Could you check a few things on this model? Use its own coordinates, in mm. A direction names the side the tool comes from. Give positions to 0.01 mm unless a question says otherwise; leave off trailing zeros. Order: outer loops, then holes, each group sorted by start corner. A loop starts at its lowest first (then second) coordinate and runs counter-clockwise, first axis right, second up.
(1) Will these pins go through, and if not, where does the flat tip stop? pin 1 (10 mm diameter, centred on x = -18, y = -38, fed in from +Z); pin 2 (2 mm diameter, centred on x = 14.5, z = 20.5, fed in from +Y); pin 3 (12 mm diameter, centred on x = 15, y = 17, fed in from -Z).
(2) On a 3-axis mill with a long thin cutter (end or side, diameter ignored), from which of +Z, -Z, +X, -X, +Y, -Y can I reach the whole of each face in a straight line? I mean faces 5 (the flat face through (40.926, -13, 13)), 6 (the flat face through (-40.074, -13, 22)), 7 (the flat face through (-38, -1.008, 17)), 8 (the flat face through (18.926, 27, 14)), 9 (the flat face through (2, -12, 27)). Say none if no direction works.
(3) If I drill on probe 1 along X at (y, z) = (-23, 36.5); probe 2 along X at (y, z) = (-33, 14.5); probe 3 along Y at (x, z) = (0, 32), over which ranges is the centre line in solid material (lowest first)?
(4) If we mould it in two halves opening along Y, with no side actions, what happens to faces 1 (the flat face through (16.926, 27, 14)), 2 (the cylindrical face through (45.02, 28.14, 22.82)), 3 (the flat face through (-9, 23.992, 13)), 4 (the flat face through (2, -51.008, 36))? For each: released by +Y, released by -Y, zero draft, split by the parting line, or undercut.
(5) Imagine slicing it at A-A, the plane x = -2. Write out the boundary of the cut face in (y, z), then the cut area to 3 significant figures.
(6) Imagine slicing it at C-C, the plane y = -26. Write out the boundary of the cut face in (x, z).
(7) Imagine slicing it at B-B, the plane y = 13. Write out the boundary of the cut face in (x, z), then the cut area to 3 significant figures.
(8) Imagine slicing it at D-D, the plane x = -15. Write out the boundary of the cut face in (y, z), then the cut area to 3 significant figures.
from build123d import *

# Parameters (mm, degrees)
ESQUISSE1_W             = 86
ESQUISSE1_H             = 83
BOSS_EXTRU_1_DEPTH      = 45
ESQUISSE2_W             = 82
ESQUISSE2_H             = 79
ENL_V_MAT_EXTRU_1_DEPTH = 3
ESQUISSE3_W             = 76
ESQUISSE3_H             = 73
ENL_V_MAT_EXTRU_2_DEPTH = 20
ESQUISSE5_W             = 80
ESQUISSE5_H             = 77
ENL_V_MAT_EXTRU_3_DEPTH = 18
ESQUISSE7_W             = 20
ESQUISSE7_H             = 16
ENL_V_MAT_EXTRU_4_DEPTH = 18
ESQUISSE8_W             = 20
ESQUISSE8_H             = 16
ENL_V_MAT_EXTRU_5_DEPTH = 18
ESQUISSE10_W            = 10
ESQUISSE10_H            = 25
ENL_V_MAT_EXTRU_6_DEPTH = 18
ESQUISSE12_R            = 0.5
ENL_V_MAT_EXTRU_9_DEPTH = 18
CONG_2_R                = 3


with BuildPart() as part:
    # Esquisse1 → Boss.-Extru.1 (new body)
    with BuildSketch(Plane.XY):
        with Locations((2.925773196, -12.508247423)):
            Rectangle(ESQUISSE1_W, ESQUISSE1_H)
    extrude(amount=BOSS_EXTRU_1_DEPTH)

    # Esquisse2 → Enlèv. mat.-Extru.1 (cut)
    with BuildSketch(Plane(origin=(0, 0, 0), x_dir=(-1, 0, 0), z_dir=(0, 0, -1))):
        with Locations((-2.925773196, -12.508247423)):
            Rectangle(ESQUISSE2_W, ESQUISSE2_H)
    extrude(amount=-ENL_V_MAT_EXTRU_1_DEPTH, mode=Mode.SUBTRACT)

    # Esquisse3 → Enlèv. mat.-Extru.2 (cut)
    with BuildSketch(Plane(origin=(0, 0, 3), x_dir=(-1, 0, 0), z_dir=(0, 0, -1))):
        with Locations((-2.925773196, -12.508247423)):
            Rectangle(ESQUISSE3_W, ESQUISSE3_H)
    extrude(amount=-ENL_V_MAT_EXTRU_2_DEPTH, mode=Mode.SUBTRACT)

    # Esquisse5 → Enlèv. mat.-Extru.3 (cut)
    with BuildSketch(Plane.XY.offset(45)):
        with Locations((2.925773196, -12.508247423)):
            Rectangle(ESQUISSE5_W, ESQUISSE5_H)
    extrude(amount=-ENL_V_MAT_EXTRU_3_DEPTH, mode=Mode.SUBTRACT)

    # Esquisse7 → Enlèv. mat.-Extru.4 (cut)
    with BuildSketch(Plane(origin=(0, 28.991752577, 0), x_dir=(1, 0, 0), z_dir=(0, 1, 0))):
        with Locations((28.925773196, -14)):
            Rectangle(ESQUISSE7_W, ESQUISSE7_H)
    extrude(amount=-ENL_V_MAT_EXTRU_4_DEPTH, mode=Mode.SUBTRACT)

    # Esquisse8 → Enlèv. mat.-Extru.5 (cut)
    with BuildSketch(Plane(origin=(0, 28.991752577, 0), x_dir=(1, 0, 0), z_dir=(0, 1, 0))):
        with Locations((6.925773196, -14)):
            Rectangle(ESQUISSE8_W, ESQUISSE8_H)
    extrude(amount=-ENL_V_MAT_EXTRU_5_DEPTH, mode=Mode.SUBTRACT)

    # Esquisse10 → Enlèv. mat.-Extru.6 (cut)
    with BuildSketch(Plane.ZY.offset(40.074226804)):
        with Locations((17, 11.491752577)):
            Rectangle(ESQUISSE10_W, ESQUISSE10_H)
    extrude(amount=-ENL_V_MAT_EXTRU_6_DEPTH, mode=Mode.SUBTRACT)

    # Esquisse12 → Enlèv. mat.-Extru.9 (cut)
    with BuildSketch(Plane.ZY.offset(40.074226804)):
        with Locations((29, 3.991752577)):
            Circle(ESQUISSE12_R)
    extrude(amount=-ENL_V_MAT_EXTRU_9_DEPTH, mode=Mode.SUBTRACT)

    # Congé2
    cong_2_edges = [part.edges().sort_by_distance(p)[0] for p in [
        (-40.074226804, 28.991752577, 22.5),
        (45.925773196, 28.991752577, 22.5),
        (45.925773196, -54.008247423, 22.5),
        (-40.074226804, -54.008247423, 22.5),
    ]]
    fillet(cong_2_edges, radius=CONG_2_R)


solid = part.part
Answer block:
1. pin 1: stops at z = 27
1. pin 2: stops at y = -49.01
1. pin 3: stops at z = 23
2. face 5: -Z
2. face 6: +Z, -Z, -X, +Y, -Y
2. face 7: -X
2. face 8: +Y
2. face 9: +Z
3. probe 1: x = -40.07 to -37.07, 42.93 to 45.93
3. probe 2: x = -40.07 to -35.07, 40.93 to 45.93
3. probe 3: y = -54.01 to -51.01, 25.99 to 28.99
4. face 1: zero draft
4. face 2: released by +Y
4. face 3: undercut
4. face 4: undercut
5. outline: (-54.01, 0) - (-52.01, 0) - (-52.01, 3) - (-49.01, 3) - (-49.01, 23) - (23.99, 23) - (23.99, 22) - (28.99, 22) - (28.99, 45) - (25.99, 45) - (25.99, 27) - (-51.01, 27) - (-51.01, 45) - (-54.01, 45) - close; (23.99, 3) - (26.99, 3) - (26.99, 0) - (28.99, 0) - (28.99, 6) - (23.99, 6) - close
5. area: 572 mm2
6. outline: (-40.07, 0) - (-38.07, 0) - (-38.07, 3) - (-35.07, 3) - (-35.07, 23) - (40.93, 23) - (40.93, 3) - (43.93, 3) - (43.93, 0) - (45.93, 0) - (45.93, 45) - (42.93, 45) - (42.93, 27) - (-37.07, 27) - (-37.07, 45) - (-40.07, 45) - close
7. outline: (-40.07, 0) - (-38.07, 0) - (-38.07, 3) - (-35.07, 3) - (-35.07, 12) - (-40.07, 12) - close; (-40.07, 22) - (-35.07, 22) - (-35.07, 23) - (40.93, 23) - (40.93, 3) - (43.93, 3) - (43.93, 0) - (45.93, 0) - (45.93, 45) - (42.93, 45) - (42.93, 27) - (-37.07, 27) - (-37.07, 45) - (-40.07, 45) - close
7. area: 614 mm2
8. outline: (-54.01, 0) - (-52.01, 0) - (-52.01, 3) - (-49.01, 3) - (-49.01, 23) - (23.99, 23) - (23.99, 3) - (26.99, 3) - (26.99, 0) - (28.99, 0) - (28.99, 45) - (25.99, 45) - (25.99, 27) - (-51.01, 27) - (-51.01, 45) - (-54.01, 45) - close
8. area: 652 mm2
